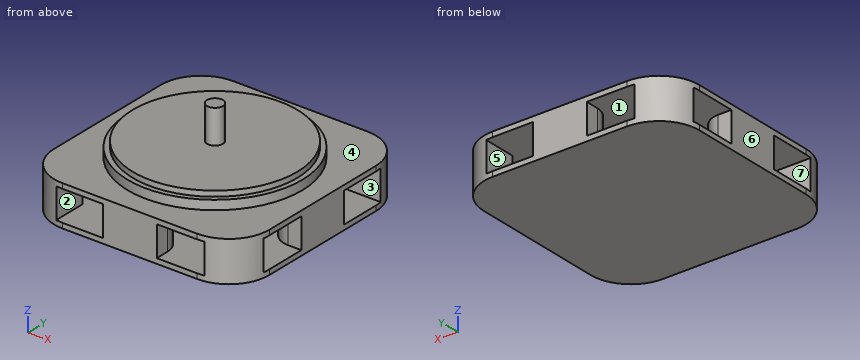
from build123d import *

# Parameters (mm, degrees)
F0_R         = 311.15
F1_DEPTH     = 20.574
F2_R         = 330.2
F3_DEPTH     = 35.052
F4_W         = 812.8
F4_H         = 812.8
F5_DEPTH     = 152.4
F6_W         = 177.8
F6_H         = 114.3
F7_DEPTH     = 812.801
F8_W         = 177.8
F8_H         = 114.3
F9_DEPTH     = 812.801
F10_T1_DEPTH = 914.4
F11_R        = 76.2
F12_R        = 30.1625
F13_DEPTH    = 127


# Not quite as in the source:
# - a fillet or chamfer that OpenCascade refuses, or shapes differently, is made with other operations: its cross-section is extruded or revolved along the edge and cut away or added


with BuildPart() as f1:
    # F0 (on Top) → F1 (new body)
    with BuildSketch(Plane.XY):
        Circle(F0_R)
    extrude(amount=F1_DEPTH)

    # F2 (on face) → F3 (join)
    with BuildSketch(Plane(origin=(0, 0, 0), x_dir=(1, 0, 0), z_dir=(0, 0, -1))):
        Circle(F2_R)
    extrude(amount=F3_DEPTH)

    # F4 (on face) → F5 (join)
    with BuildSketch(Plane(origin=(0, 0, -35.052), x_dir=(1, 0, 0), z_dir=(0, 0, -1))):
        Rectangle(F4_W, F4_H)
    extrude(amount=F5_DEPTH)

    # F6 (on face) → F7 (cut, through all)
    with BuildSketch(Plane(origin=(0, 406.4, 0), x_dir=(-1, 0, 0), z_dir=(0, 1, 0))):
        with Locations((190.5, -111.252)):
            Rectangle(F6_W, F6_H)
        with Locations((-190.5, -111.252)):
            Rectangle(F6_W, F6_H)
    extrude(amount=-F7_DEPTH, mode=Mode.SUBTRACT)

    # F8 (on face) → F9 (cut, through all)
    with BuildSketch(Plane(origin=(-406.4, 0, 0), x_dir=(0, -1, 0), z_dir=(-1, 0, 0))):
        with Locations((190.5, -111.252)):
            Rectangle(F8_W, F8_H)
        with Locations((-190.5, -111.252)):
            Rectangle(F8_W, F8_H)
    extrude(amount=-F9_DEPTH, mode=Mode.SUBTRACT)

    # F10: fillet of radius 152.4 on 4 edges, made by hand

    # F10_s2 → F10_t1 (cut)
    with BuildSketch(Plane.XY.offset(-568.452)):
        with BuildLine():
            ThreePointArc((-254, -406.4), (-361.7630734528, -361.7630734528), (-406.4, -254))
            Line((-406.4, -254), (-406.4, -406.4))
            Line((-406.4, -406.4), (-254, -406.4))
        make_face()
        with BuildLine():
            ThreePointArc((-254, 406.4), (-361.7630734528, 361.7630734528), (-406.4, 254))
            Line((-406.4, 254), (-406.4, 406.4))
            Line((-406.4, 406.4), (-254, 406.4))
        make_face()
        with BuildLine():
            ThreePointArc((406.4, 254), (361.7630734528, 361.7630734528), (254, 406.4))
            Line((254, 406.4), (406.4, 406.4))
            Line((406.4, 406.4), (406.4, 254))
        make_face()
        with BuildLine():
            ThreePointArc((406.4, -254), (361.7630734528, -361.7630734528), (254, -406.4))
            Line((254, -406.4), (406.4, -406.4))
            Line((406.4, -406.4), (406.4, -254))
        make_face()
    extrude(amount=F10_T1_DEPTH, mode=Mode.SUBTRACT)

    # F11
    f11_edges = [f1.edges().sort_by_distance(p)[0] for p in [
        (279.4, -101.6, -111.252),
        (279.4, 101.6, -111.252),
        (101.6, 279.4, -111.252),
        (-101.6, 279.4, -111.252),
        (-279.4, 101.6, -111.252),
        (-279.4, -101.6, -111.252),
        (-101.6, -279.4, -111.252),
        (101.6, -279.4, -111.252),
    ]]
    fillet(f11_edges, radius=F11_R)

    # F12 (on face) → F13 (join)
    with BuildSketch(Plane.XY.offset(20.574)):
        Circle(F12_R)
    extrude(amount=F13_DEPTH)


solid = f1.part
Work out the finished part from the listing and answer in its coordinate system (mm). Face numbers are marked on the shaded views. A direction names the side the tool comes from. Give positions to 0.01 mm unless a question says otherwise; leave off trailing zeros. Order: outer loops, then holes, each group sorted by start corner. A loop starts at its lowest first (then second) coordinate and runs counter-clockwise, first axis right, second up. Notation, with made-up numbers: M 84.5,34.25 L 122.5,34.25 A31 ccw 122.5,71.25 Z; hole C 24,87 d10. An arc over 180 degrees is marked long. Return JSON: item names as keys, results as strings.
Q1. Find section D-D, the plane y = 127. Write down the section's boundary in (x, z).
Answer below:
{"outline": "M -406.4,-187.45 L 406.4,-187.45 L 406.4,-168.4 L -406.4,-168.4 Z; M -406.4,-54.1 L 406.4,-54.1 L 406.4,-35.05 L 304.8,-35.05 L 304.8,0 L 284.05,0 L 284.05,20.57 L -284.05,20.57 L -284.05,0 L -304.8,0 L -304.8,-35.05 L -406.4,-35.05 Z"}
Q2. Which of the six approach directions +Z, -Z, +X, -X, +Y, -Y give full straight-line access (tool end or side, diameter ignored) to the marked faces 1, 2, 3 and 4?
Answer below:
{"face 1": "none", "face 2": "+Y, -Y", "face 3": "+X, -X", "face 4": "+Z"}
Q3. The mould has two halves that part along X. Classify the marked faces 5, 6 and 7: pulls with the +X half, pulls with the -X half, needs draft (parallel to the pull), parting line crosses it, or undercut.
Answer below:
{"face 5": "undercut", "face 6": "pulls with the -X half", "face 7": "needs draft"}
Q4. Find the intervals of material crossed by line 1 along X through (y, z) = (21, -132); line 2 along Z through (x, y) = (-172, 108.5), in increasing order. Write a range as [from, to].
Answer below:
{"line 1": "x = [-406.4, -279.4], [-101.6, 101.6], [279.4, 406.4]", "line 2": "z = [-187.45, -168.4], [-54.1, 20.57]"}
Q5. Find section C-C, the plane z = -100. State how many separate pieces and enclosed holes the cut face has, and give its area (3 significant figures).
Answer below:
{"separate pieces": "9", "enclosed holes": "0", "area": "179,000 mm^2"}
Q6. Find section A-A, the plane y = 0. Write down the section's boundary in (x, z), and give its area (3 significant figures).
Answer below:
{"outline": "M -406.4,-187.45 L 406.4,-187.45 L 406.4,-35.05 L 330.2,-35.05 L 330.2,0 L 311.15,0 L 311.15,20.57 L 30.16,20.57 L 30.16,147.57 L -30.16,147.57 L -30.16,20.57 L -311.15,20.57 L -311.15,0 L -330.2,0 L -330.2,-35.05 L -406.4,-35.05 Z; hole M -279.4,-168.4 L -101.6,-168.4 L -101.6,-54.1 L -279.4,-54.1 Z; hole M 101.6,-168.4 L 279.4,-168.4 L 279.4,-54.1 L 101.6,-54.1 Z", "area": "127,000 mm^2"}
Q7. Each of these flat-tipped pins is pushed along its axis until it touches: pin 1 (15 mm diameter, centred on x = 378, z = -122, fed in from +Y); pin 2 (4 mm diameter, centred on y = -281, z = -90, fed in from +X); pin 3 (1.5 mm diameter, centred on y = 180, z = 0.5, fed in from +X). Where does it stop, or does it pass through?
Answer below:
{"pin 1": "stops at y = 352.25", "pin 2": "stops at x = 404.27", "pin 3": "stops at x = 277.19"}
